Part model, mm, in its own coordinate system. A direction names the side the tool comes from. Give positions to 0.01 mm unless a question says otherwise; leave off trailing zeros. Order: outer loops, then holes, each group sorted by start corner. A loop starts at its lowest first (then second) coordinate and runs counter-clockwise, first axis right, second up. Notation, with made-up numbers: (34, 47.5) -> (78, 47.5) arc R24 cw to (78, 62.5) -> close; hole circle Ø4 at (74.25, 69.25). An arc over 180 degrees is marked (long way). Write item = value, one per line. Start each with the question number.
Item 1: Pull direction X, two halves, no side cores. Call faces 1 (the face through (-40, -1, 0)), 2 (the face through (39, -1, -5)), 3 (the face through (20, -1, 25)): +X half, -X half, draft (parallel to the pull), parting line (faces both ways), or undercut.
Item 2: Drill centre lines: line 1 along X through (y, z) = (-1.75, -24.5); line 2 along Z through (x, y) = (-20, -1.25); line 3 along X through (y, z) = (-1.65, 2). Where is each one in solid material? Low to high.
Item 3: Tool access for faces 4 (the face through (-38, -1, -16)), 5 (the face through (38, -1, -16)), 6 (the face through (-20, -1, -23)), 7 (the face through (38, -1, 16)): list every direction of +Z, -Z, +X, -X, +Y, -Y with a clear straight run to the whole face (end or side of a thin tool).
Item 4: Band-saw the part on A-A on x = -21.5. Write the cut outline in (y, z).
Item 5: Band-saw the part on B-B on z = 4. Write the cut outline in (x, y), plus the area to 3 significant figures.
Item 6: Band-saw the part on C-C on y = -1.6. Count the separate pieces of the cut face and the enclosed holes in it, plus the area to 3 significant figures.
Item 7: Flat gauge pins, fed straight in: P1, Ø5, axis at x = -30, z = -19, coming from the +Y side; P2, Ø0.6, axis at y = -1.5, z = -19.5, coming from the -X side. Where does each tip first touch, or does it go through?
Item 8: Band-saw the part on D-D on z = -14. Write the cut outline in (x, y), plus the area to 3 significant figures.
Solid Edge part; units mm, degrees
sketch "Sketch1" plane through (0, 0, 0) normal (0, -1, 0) x (1, 0, 0)
  line L0 (40, -27) -> (40, 27)
  line L1 (40, 27) -> (-40, 27)
  line L2 (-40, 27) -> (-40, -27)
  line L3 (-40, -27) -> (40, -27)
extrude "Protrusion1" add sketch "Sketch1" along normal blind 2
sketch "Sketch2" plane through (0, 0, 0) normal (0, -1, 0) x (1, 0, 0)
  line L0 (-25, 23) -> (-15, 23)
  line L1 (-15, 23) -> (-15, 25)
  line L2 (-15, 25) -> (-25, 25)
  line L3 (-25, 25) -> (-25, 23)
extrude "ExtrudedCutout_1" cut sketch "Sketch2" along normal blind 2
sketch "Sketch3" plane through (0, 0, 0) normal (0, -1, 0) x (1, 0, 0)
  line L0 (25, 25) -> (15, 25)
  line L1 (15, 25) -> (15, 23)
  line L2 (15, 23) -> (25, 23)
  line L3 (25, 23) -> (25, 25)
extrude "ExtrudedCutout_2" cut sketch "Sketch3" along normal blind 2
sketch "Sketch4" plane through (0, 0, 0) normal (0, -1, 0) x (1, 0, 0)
  line L0 (15, -25) -> (25, -25)
  line L1 (25, -25) -> (25, -23)
  line L2 (25, -23) -> (15, -23)
  line L3 (15, -23) -> (15, -25)
extrude "ExtrudedCutout_3" cut sketch "Sketch4" along normal blind 2
sketch "Sketch5" plane through (0, 0, 0) normal (0, -1, 0) x (1, 0, 0)
  line L0 (-15, -23) -> (-25, -23)
  line L1 (-25, -23) -> (-25, -25)
  line L2 (-25, -25) -> (-15, -25)
  line L3 (-15, -25) -> (-15, -23)
extrude "ExtrudedCutout_4" cut sketch "Sketch5" along normal blind 2
sketch "Sketch6" plane through (0, 0, 0) normal (0, -1, 0) x (1, 0, 0)
  line L0 (-38, -27) -> (-38, -5)
  line L1 (-38, -5) -> (-40, -5)
  line L2 (-40, -5) -> (-40, -27)
  line L3 (-40, -27) -> (-38, -27)
extrude "ExtrudedCutout_5" cut sketch "Sketch6" along normal blind 2
sketch "Sketch7" plane through (0, 0, 0) normal (0, -1, 0) x (1, 0, 0)
  line L0 (-38, 5) -> (-38, 27)
  line L1 (-38, 27) -> (-40, 27)
  line L2 (-40, 27) -> (-40, 5)
  line L3 (-40, 5) -> (-38, 5)
extrude "ExtrudedCutout_6" cut sketch "Sketch7" along normal blind 2
sketch "Sketch8" plane through (0, 0, 0) normal (0, -1, 0) x (1, 0, 0)
  line L0 (38, -5) -> (38, -27)
  line L1 (38, -27) -> (40, -27)
  line L2 (40, -27) -> (40, -5)
  line L3 (40, -5) -> (38, -5)
extrude "ExtrudedCutout_7" cut sketch "Sketch8" along normal blind 2
sketch "Sketch9" plane through (0, 0, 0) normal (0, -1, 0) x (1, 0, 0)
  line L0 (38, 27) -> (38, 5)
  line L1 (38, 5) -> (40, 5)
  line L2 (40, 5) -> (40, 27)
  line L3 (40, 27) -> (38, 27)
extrude "ExtrudedCutout_8" cut sketch "Sketch9" along normal blind 2
sketch "Sketch10" plane through (0, 0, 0) normal (0, -1, 0) x (1, 0, 0)
  line L0 (-18.12, -2) -> (-8.12, -2)
  line L1 (-8.12, -2) -> (-8.12, 9)
  line L2 (-8.12, 9) -> (-18.12, 9)
  line L3 (-18.12, 9) -> (-18.12, -2)
extrude "ExtrudedCutout_9" cut sketch "Sketch10" along normal blind 2
properties material "Acrylic, high impact grade"
Values found:
q1.face_1 = -X half
q1.face_2 = draft
q1.face_3 = undercut
q2.line_1 = -38 to -25, -15 to 15, 25 to 38
q2.line_2 = -27 to -25, -23 to 23, 25 to 27
q2.line_3 = -40 to -18.12, -8.12 to 40
q3.face_4 = -Z, -X, +Y, -Y
q3.face_5 = -Z, +X, +Y, -Y
q3.face_6 = +Y, -Y
q3.face_7 = +Z, +X, +Y, -Y
q4.outline = (-2, -27) -> (0, -27) -> (0, -25) -> (-2, -25) -> close; (-2, -23) -> (0, -23) -> (0, 23) -> (-2, 23) -> close; (-2, 25) -> (0, 25) -> (0, 27) -> (-2, 27) -> close
q5.outline = (-40, -2) -> (-18.12, -2) -> (-18.12, 0) -> (-40, 0) -> close; (-8.12, -2) -> (40, -2) -> (40, 0) -> (-8.12, 0) -> close
q5.area = 140 mm^2
q6.separate_pieces = 1
q6.enclosed_holes = 5
q6.area = 3,950 mm^2
q7.P1 = 0
q7.P2 = -38
q8.outline = (-38, -2) -> (38, -2) -> (38, 0) -> (-38, 0) -> close
q8.area = 152 mm^2
